CAD build for the part. Positions are in the model's coordinates, mm. Face numbers are marked on the shaded views. A direction names the side the tool comes from. Round coordinates to 2 decimals unless told otherwise and drop trailing zeros. Loops run counter-clockwise (first coordinate to the right, second up) from the corner with the lowest first, then second, coordinate; pieces in that order, holes last. Notation, with made-up numbers: (-2, -5.5) - (27, -5.5) arc R23 cw to (27, 30.5) - close; hole circle Ø10 at (59.25, 87.25). An arc over 180 degrees is marked (long way). One line per question, with ' | ' between items.
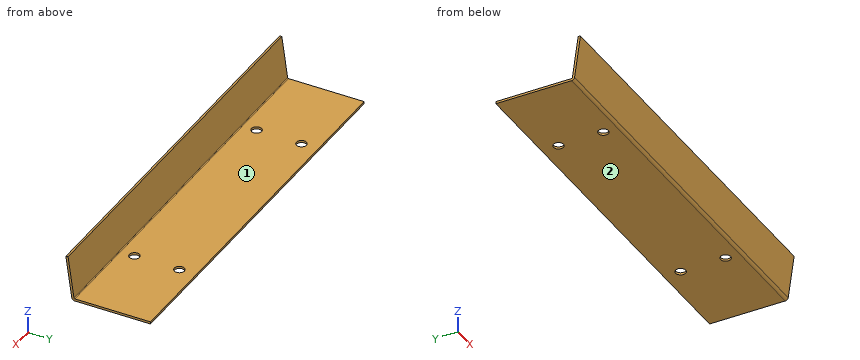
```python
from build123d import *

# Parameters (mm, degrees)
SKETCH1_W            = 350
SKETCH1_H            = 70
BASE_FLANGE1_DEPTH   = 2
EDGE_FLANGE1_START   = -175
EDGE_FLANGE1_DEPTH   = 350
EDGE_FLANGE1_2_DEPTH = 350
M8_CLEARANCE_HOLE1_D = 9


# Read off the part's stored shape, not the designer's step: Edge-Flange1
# Sheet-metal steps are written as plain solids
with BuildPart() as part:
    # Sketch1 → Base-Flange1 (new body)
    with BuildSketch(Plane.XY):
        Rectangle(SKETCH1_W, SKETCH1_H)
    extrude(amount=-BASE_FLANGE1_DEPTH)

    # Edge-Flange1 outline → Edge-Flange1 (cut)
    with BuildSketch(Plane.YZ.offset(EDGE_FLANGE1_START)):
        with BuildLine():
            ThreePointArc((-32.340028244, -2), (-33.994295453, -1.443395312), (-34.975630642, 0))
            Line((-34.975630642, 0), (-35, 0))
            Line((-35, 0), (-35, -2))
            Line((-35, -2), (-32.340028244, -2))
        make_face()
    extrude(amount=EDGE_FLANGE1_DEPTH, mode=Mode.SUBTRACT)

    # Edge-Flange1 2 outline → Edge-Flange1 2 (add)
    with BuildSketch(Plane.YZ.offset(EDGE_FLANGE1_START)):
        with BuildLine():
            Line((-40.285842369, 37.61072275), (-35.049995841, 0.355738892))
            ThreePointArc((-35.049995841, 0.355738892), (-35.018725163, 0.176633592), (-34.975630642, 0))
            Line((-34.975630642, 0), (-32.340028244, 0))
            ThreePointArc((-32.340028244, 0), (-32.823281325, 0.180680923), (-33.069459703, 0.634085094))
            Line((-33.069459703, 0.634085094), (-38.305306232, 37.889068952))
            Line((-38.305306232, 37.889068952), (-40.285842369, 37.61072275))
        make_face()
    extrude(amount=EDGE_FLANGE1_2_DEPTH)

    # M8 Clearance Hole1 (through all)
    with Locations(Plane(origin=(-100, 20, 0), x_dir=(1, 0, 0), z_dir=(0, 0, 1))):
        with Locations((0, 0), (0, -40), (200, -40), (200, 0)):
            Hole(M8_CLEARANCE_HOLE1_D / 2)


solid = part.part
```
(1) Cut at B-B, the plane y = 20. Write the cut outline in (x, z).
Results found:
outline: (-175, -2) - (-104.5, -2) - (-104.5, 0) - (-175, 0) - close; (-95.5, -2) - (95.5, -2) - (95.5, 0) - (-95.5, 0) - close; (104.5, -2) - (175, -2) - (175, 0) - (104.5, 0) - close
(2) Cut at A-A, the plane x = 100. Write the cut outline in (y, z), then the cut area to 3 significant figures.
Results found:
outline: (-40.29, 37.61) - (-35.05, 0.36) arc R2.74 ccw to (-32.34, -2) - (-24.5, -2) - (-24.5, 0) - (-32.34, 0) arc R0.74 cw to (-33.07, 0.63) - (-38.31, 37.89) - close; (-15.5, -2) - (15.5, -2) - (15.5, 0) - (-15.5, 0) - close; (24.5, -2) - (35, -2) - (35, 0) - (24.5, 0) - close | area: 179 mm²
(3) Probe L1, parallel to Y at x = 100, z = -1.3; L2, parallel to Z at x = 156.5, y = 19.5; L3, parallel to Y at x = -100, z = -1.15. List the from-to ranges inside material, lowest first.
Results found:
L1: y = -34.17 to -24.5, -15.5 to 15.5, 24.5 to 35 | L2: z = -2 to 0 | L3: y = -34.32 to -24.5, -15.5 to 15.5, 24.5 to 35
(4) Cut at C-C, the plane x = -110. Write the cut outline in (y, z).
Results found:
outline: (-40.29, 37.61) - (-35.05, 0.36) arc R2.74 ccw to (-32.34, -2) - (35, -2) - (35, 0) - (-32.34, 0) arc R0.74 cw to (-33.07, 0.63) - (-38.31, 37.89) - close
(5) Tool access for the marked faces 1 and 2: list every direction of +Z, -Z, +X, -X, +Y, -Y with a clear straight run to the whole face (end or side of a thin tool).
Results found:
face 1: +Z, +X, -X, +Y | face 2: -Z, +X, -X, +Y, -Y
(6) Drop flat-ended pins along their axis: P1, Ø10, axis at x = 119, z = 13, coming from the -Y side; P2, Ø8, axis at x = -100, y = 20, coming from the -Z side; P3, Ø1.5, axis at x = -111.5, z = 4, coming from the -Y side; P4, Ø11.5, axis at x = -100, y = -20, coming from the -Z side. Give the stop position or say it passes through.
Results found:
P1: stops at y = -37.53 | P2: passes through | P3: stops at y = -35.67 | P4: stops at z = -2
(7) Cut at D-D, the plane z = 17. Write the cut outline in (x, y), then the cut area to 3 significant figures.
Results found:
outline: (-175, -37.39) - (175, -37.39) - (175, -35.37) - (-175, -35.37) - close | area: 707 mm²
